For this review, use the dimensioned drawing (mm, ordinates from the lowest corner) and the shaded views. A direction names the side the tool comes from. Coordinates: 2 decimals unless noted, no trailing zeros. Loops run counter-clockwise (first coordinate to the right, second up) from the corner with the lowest first, then second, coordinate; pieces in that order, holes last. Notation, with made-up numbers: (-6, 41) - (-1, 41) arc R16 cw to (-1, 60) - close; hole circle Ø4 at (32, 0). An arc over 180 degrees is marked (long way). Answer in a Markdown table with one row per item. Add a question column.
(1) Machinability: for the marked faces 1, 2 and 3, which of the approach directions +Z, -Z, +X, -X, +Y, -Y give a long, thin tool a straight path to every point of the face, cutting with its end or side? Answer none if there is none.
(2) We need section B-B on x = 14.25. Write out the cut boundary in (y, z), plus the area to 3 significant figures.
(3) For P1, Ø1.9, axis at x = 15, z = 3, coming from the +Y side; P2, Ø0.5, axis at x = 15, y = 3.5, coming from the +Z side, all flat-tipped, find the tip position at first contact; note any pin that passes through.
(4) For line 1 along Z through (x, y) = (12, 3.2); line 2 along X through (y, z) = (0.65, 2.7); line 3 along Y through (x, z) = (1.5, 0.65), list the stretches that pass through material, from the lowest coordinate up.
(5) We need section A-A on z = 1.7. Write out the cut boundary in (x, y), plus the area to 3 significant figures.
(6) We need section C-C on y = 2.15. Write out the cut boundary in (x, z).
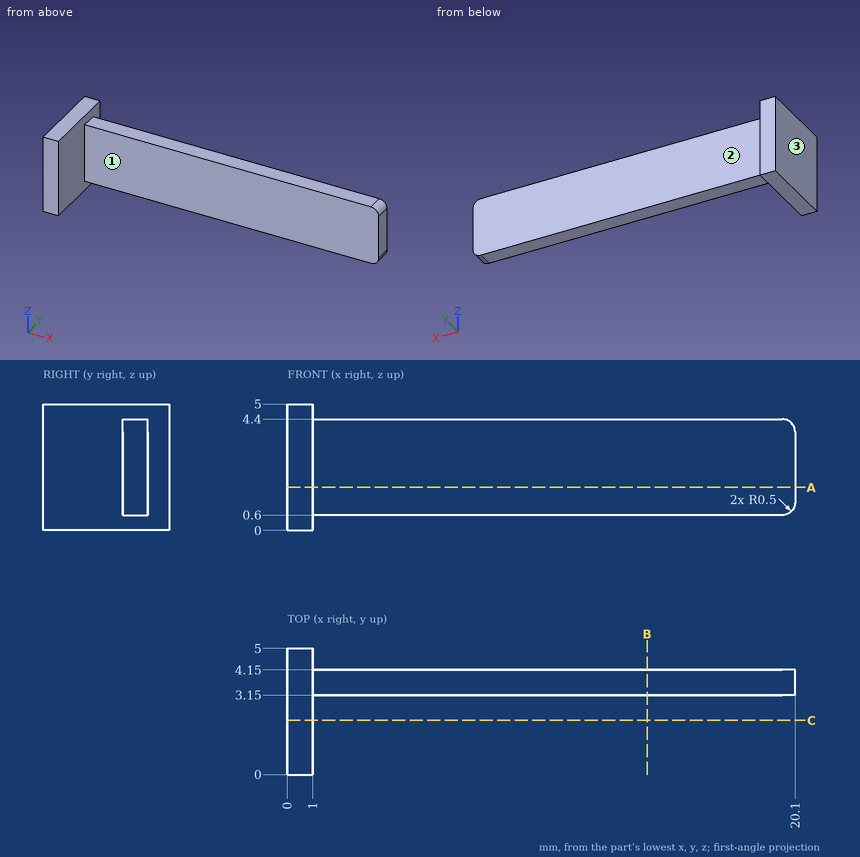
Outcome:
| question | item | result |
|---|---|---|
| 1 | face 1 | +Z, -Z, +X, -Y |
| 1 | face 2 | +Z, -Z, +X, +Y |
| 1 | face 3 | +Z, -Z, -X, +Y, -Y |
| 2 | outline | (3.15, 0.6) - (4.15, 0.6) - (4.15, 4.4) - (3.15, 4.4) - close |
| 2 | area | 3.80 mm² |
| 3 | P1 | y = 4.15 |
| 3 | P2 | z = 4.4 |
| 4 | line 1 | 0.6 to 4.4 |
| 4 | line 2 | 0 to 1 |
| 4 | line 3 | 3.15 to 4.15 |
| 5 | outline | (0, 0) - (1, 0) - (1, 3.15) - (20.1, 3.15) - (20.1, 4.15) - (1, 4.15) - (1, 5) - (0, 5) - close |
| 5 | area | 24.1 mm² |
| 6 | outline | (0, 0) - (1, 0) - (1, 5) - (0, 5) - close |
